Part model, mm, in its own coordinate system. Face numbers are marked on the shaded views. Round coordinates to 2 decimals unless told otherwise and drop trailing zeros. Write each loop counter-clockwise with the first axis right and the second up, starting at its lowest first coordinate (ties: lowest second). Pieces come first, ordered by that corner, then holes. Notation, with made-up numbers: (-29, 45.5) -> (-3, 45.5) arc R15 ccw to (-3, 60.5) -> close; hole circle Ø2 at (47, 63). An arc over 180 degrees is marked (long way). Return JSON: item names as keys, results as strings. Group by question number.
```python
from build123d import *

# Parameters (mm, degrees)
F0_R     = 11.049
F0_R_2   = 11.05
F1_DEPTH = 7
F2_SIZE  = 2.032


# Not quite as in the source:
# - a feature names something its author has since deleted; it is built from what else it names


with BuildPart() as f1:
    # F0 (on Top) → F1 (new body)
    with BuildSketch(Plane.XY):
        with BuildLine():
            ThreePointArc((-8.7042735718, 22.0943097642), (-12.2328176499, 5.8189544339), (-24.7131356106, -5.2073540163))
            ThreePointArc((-24.7131356106, -5.2073540163), (-17.821671092, -10.084264276), (-14.930456808, -18.0163142542))
            ThreePointArc((-14.930456808, -18.0163142542), (0.0145480917, -13.5128951169), (14.9256967567, -18.1271773868))
            ThreePointArc((14.9256967567, -18.1271773868), (17.7880815001, -10.1284239204), (24.7131356106, -5.2073540163))
            ThreePointArc((24.7131356106, -5.2073540163), (12.1415366781, 5.9758444424), (8.7441728022, 22.4551328426))
            ThreePointArc((8.7441728022, 22.4551328426), (0.0821273079, 19.2679731194), (-8.7042735718, 22.0943097642))
        make_face()
        Circle(F0_R, mode=Mode.SUBTRACT)
        with BuildLine():
            ThreePointArc((-14.930456808, -18.0163142542), (-17.821671092, -10.084264276), (-24.7131356106, -5.2073540163))
            ThreePointArc((-24.7131356106, -5.2073540163), (-40.5273347614, -27.0082695647), (-14.9149335915, -18.6791807883))
            ThreePointArc((-14.9149335915, -18.6791807883), (-14.9188149276, -18.3476566518), (-14.930456808, -18.0163142542))
        make_face()
        with Locations((-29.0754335915, -18.6791807883)):
            Circle(F0_R_2, mode=Mode.SUBTRACT)
        with BuildLine():
            ThreePointArc((13.9525783408, 33.428221941), (-6.5471611927, 46.095014193), (-8.7042735718, 22.0943097642))
            ThreePointArc((-8.7042735718, 22.0943097642), (0.0821273079, 19.2679731194), (8.7441728022, 22.4551328426))
            ThreePointArc((8.7441728022, 22.4551328426), (12.5843929813, 27.3549984844), (13.9525783408, 33.428221941))
        make_face()
        with Locations((-0.2106978791, 33.428221941)):
            Circle(F0_R_2, mode=Mode.SUBTRACT)
        with BuildLine():
            ThreePointArc((24.7131356106, -5.2073540163), (17.7880815001, -10.1284239204), (14.9256967567, -18.1271773868))
            ThreePointArc((14.9256967567, -18.1271773868), (28.7993794297, -32.8369897413), (43.2359335915, -18.6791807883))
            ThreePointArc((43.2359335915, -18.6791807883), (37.404522368, -7.2272796184), (24.7131356106, -5.2073540163))
        make_face()
        with Locations((29.0754335915, -18.6791807883)):
            Circle(F0_R_2, mode=Mode.SUBTRACT)
    extrude(amount=F1_DEPTH)

    # F2
    f2_edges = [f1.edges().sort_by_distance(p)[0] for p in [
        (-12.232818, 5.818954, 7),
        (12.141537, 5.975844, 7),
        (0.014548, -13.512895, 7),
        (0.014548, -13.512895, 0),
        (12.141537, 5.975844, 0),
        (-12.232818, 5.818954, 0),
        (-40.329196, -27.274097, 0),
        (40.362786, -27.229938, 0),
        (-0.503523, 47.588471, 0),
        (-40.329196, -27.274097, 7),
        (40.362786, -27.229938, 7),
        (-0.503523, 47.588471, 7),
    ]]
    chamfer(f2_edges, length=F2_SIZE)


solid = f1.part
```
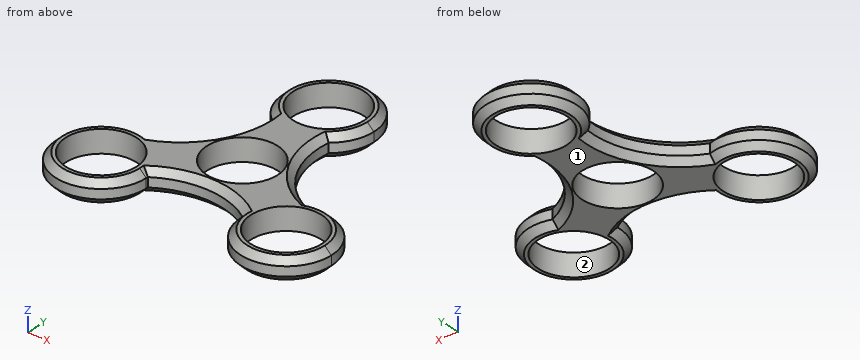
Item 1: Cut at A-A (z = 4). Write the cut outline in (x, y).
Item 2: Wall check: L1, parallel to Y at x = 0, z = 4.75; L2, parallel to Y at x = 0, z = 5.75; L3, parallel to X at y = -18, z = 6.25. Give the ranges that are in metal, low to high.
Item 3: Cut at B-B (x = 2.5). State how many separate pieces and enclosed holes the cut face has, then the cut area to 3 significant figures.
Item 4: Two-plate mould, pull along Y, no slides. Class the marked faces 1 and 2: released by +Y, released by -Y, zero draft, split by the parting line, or undercut.
Item 5: Flat gauge pins, fed straight in: P1, Ø20, axis at x = -0.21, y = 33.43, coming from the +Z side; P2, Ø2, axis at x = -18, y = -1, coming from the +Z side; P3, Ø2, axis at y = -11.5, z = 5.5, coming from the -X side. Where does each tip first touch, or does it go through?
Checks:
{
 "1": {"outline": "(-24.71, -5.21) arc R14.16 ccw (long way) to (-14.93, -18.02) arc R26.72 cw to (14.93, -18.13) arc R14.16 ccw (long way) to (24.71, -5.21) arc R26.73 cw to (8.74, 22.46) arc R14.16 ccw (long way) to (-8.7, 22.09) arc R26.73 cw to start; hole circle Ø22.1 at (-29.08, -18.68); hole circle Ø22.1 at (-0.21, 33.43); hole circle Ø22.1 at (0, 0); hole circle Ø22.1 at (29.08, -18.68)"},
 "2": {"L1": "y = -13.51 to -11.05, 11.05 to 22.38, 44.48 to 47.59", "L2": "y = -12.73 to -11.05, 11.05 to 22.38, 44.48 to 46.81", "L3": "x = -41.94 to -40.1, -18.05 to -16.21, 16.21 to 18.05, 40.1 to 41.94"},
 "3": {"separate pieces": "3", "enclosed holes": "0", "area": "118 mm2"},
 "4": {"face 1": "zero draft", "face 2": "undercut"},
 "5": {"P1": "passes through", "P2": "stops at z = 5.93", "P3": "stops at x = -41.74"}
}
